Here's how the part is built. I have some questions about the finished solid (model axes, mm). Round coordinates to 2 decimals unless told otherwise and drop trailing zeros. Write each loop counter-clockwise with the first axis right and the second up, starting at its lowest first coordinate (ties: lowest second). Pieces come first, ordered by that corner, then holes. Notation, with made-up numbers: (78, 19) -> (116, 19) arc R24 cw to (116, 31) -> close; hole circle Ø10 at (71.25, -25.5). An arc over 180 degrees is marked (long way). Answer in a Markdown table with one row per item. Add a question column.
Autodesk Inventor part; units mm, degrees
ref_plane "att_plate_magnet_XY" through (19.5, -5, 7.5) normal (0, 0, 1) x (1, 0, 0)
ref_plane "att_plate_magnet_YZ" through (19.5, -5, 7.5) normal (1, 0, 0) x (0, 1, 0)
ref_plane "att_plate_magnet_ZX" through (19.5, -5, 7.5) normal (0, 1, 0) x (0, 0, 1)
sketch "Sketch_14" plane through (0, 0, 0) normal (0, 1, 0) x (-1, 0, 0)
  line L0 (25.5, 7.5) -> (-25.5, 7.5)
  line L1 (-25.5, 7.5) -> (-25.5, -7.5)
  line L2 (-25.5, -7.5) -> (25.5, -7.5)
  line L3 (25.5, -7.5) -> (25.5, 7.5)
  circle A0 centre (-15.5, -2.5) radius 2.75
  circle A1 centre (15.5, -2.5) radius 2.75
extrude "Extrusion1" add sketch "Sketch_14" along normal mid plane 20
sketch "Sketch_2" plane through (19.5, 0, 0) normal (1, 0, 0) x (0, 0, -1)
  line L0 (7.5, -5) -> (-7.5, -5)
  line L1 (-7.5, -5) -> (-7.5, -3)
  line L2 (-7.5, -3) -> (-7.121, -3.379)
  line L3 (-7.121, -3.379) -> (7.121, -3.379)
  line L4 (7.121, -3.379) -> (7.5, -3)
  line L5 (7.5, -3) -> (7.5, -5)
  line L6 (7.5, -5) -> (-7.5, -5)
revolve "Revolution1" cut sketch "Sketch_2" angle 360 about axis through (19.5, -5, -7.5) along (0, 0, -1)
thread "Thread1"
sketch "Sketch_3" plane through (-19.5, 0, 0) normal (1, 0, 0) x (0, 0, -1)
  line L0 (7.5, -5) -> (-7.5, -5)
  line L1 (-7.5, -5) -> (-7.5, -3)
  line L2 (-7.5, -3) -> (-7.121, -3.379)
  line L3 (-7.121, -3.379) -> (7.121, -3.379)
  line L4 (7.121, -3.379) -> (7.5, -3)
  line L5 (7.5, -3) -> (7.5, -5)
  line L6 (7.5, -5) -> (-7.5, -5)
revolve "Revolution2" cut sketch "Sketch_3" angle 360 about axis through (-19.5, -5, -7.5) along (0, 0, -1)
thread "Thread2"
ref_plane "att_plate_magnet_XY" through (19.5, -5, 7.5) normal (0, 0, 1) x (1, 0, 0)
ref_plane "att_plate_magnet_YZ" through (19.5, -5, 7.5) normal (1, 0, 0) x (0, 1, 0)
ref_plane "att_plate_magnet_ZX" through (19.5, -5, 7.5) normal (0, 1, 0) x (0, 0, 1)
ref_plane "to_magnetT_XY" through (-19.5, -5, 7.5) normal (0, 0, 1) x (1, 0, 0)
ref_plane "to_magnetT_YZ" through (-19.5, -5, 7.5) normal (1, 0, 0) x (0, 1, 0)
ref_plane "to_magnetT_ZX" through (-19.5, -5, 7.5) normal (0, 1, 0) x (0, 0, 1)
ref_plane "c1_XY" through (-15.5, 10, -2.5) normal (0, 1, 0) x (1, 0, 0)
ref_plane "c1_YZ" through (-15.5, 10, -2.5) normal (1, 0, 0) x (0, 0, -1)
ref_plane "c1_ZX" through (-15.5, 10, -2.5) normal (0, 0, -1) x (0, 1, 0)
ref_plane "c2_XY" through (15.5, 10, -2.5) normal (0, 1, 0) x (1, 0, 0)
ref_plane "c2_YZ" through (15.5, 10, -2.5) normal (1, 0, 0) x (0, 0, -1)
ref_plane "c2_ZX" through (15.5, 10, -2.5) normal (0, 0, -1) x (0, 1, 0)
ref_plane "c3_XY" through (-15.5, -10, -2.5) normal (0, 1, 0) x (1, 0, 0)
ref_plane "c3_YZ" through (-15.5, -10, -2.5) normal (1, 0, 0) x (0, 0, -1)
ref_plane "c3_ZX" through (-15.5, -10, -2.5) normal (0, 0, -1) x (0, 1, 0)
ref_plane "c4_XY" through (15.5, -10, -2.5) normal (0, 1, 0) x (1, 0, 0)
ref_plane "c4_YZ" through (15.5, -10, -2.5) normal (1, 0, 0) x (0, 0, -1)
ref_plane "c4_ZX" through (15.5, -10, -2.5) normal (0, 0, -1) x (0, 1, 0)
ref_plane "cc3_XY" through (-15.5, 10, -2.5) normal (0, 1, 0) x (1, 0, 0)
ref_plane "cc3_YZ" through (-15.5, 10, -2.5) normal (1, 0, 0) x (0, 0, -1)
ref_plane "cc3_ZX" through (-15.5, 10, -2.5) normal (0, 0, -1) x (0, 1, 0)
ref_plane "cc4_XY" through (15.5, 10, -2.5) normal (0, 1, 0) x (1, 0, 0)
ref_plane "cc4_YZ" through (15.5, 10, -2.5) normal (1, 0, 0) x (0, 0, -1)
ref_plane "cc4_ZX" through (15.5, 10, -2.5) normal (0, 0, -1) x (0, 1, 0)
ref_plane "cc1_XY" through (-15.5, -10, -2.5) normal (0, 1, 0) x (1, 0, 0)
ref_plane "cc1_YZ" through (-15.5, -10, -2.5) normal (1, 0, 0) x (0, 0, -1)
ref_plane "cc1_ZX" through (-15.5, -10, -2.5) normal (0, 0, -1) x (0, 1, 0)
ref_plane "cc2_XY" through (15.5, -10, -2.5) normal (0, 1, 0) x (1, 0, 0)
ref_plane "cc2_YZ" through (15.5, -10, -2.5) normal (1, 0, 0) x (0, 0, -1)
ref_plane "cc2_ZX" through (15.5, -10, -2.5) normal (0, 0, -1) x (0, 1, 0)
ref_plane "d1_XY" through (15.5, 15, -5) normal (0, 1, 0) x (1, 0, 0)
ref_plane "d1_YZ" through (15.5, 15, -5) normal (1, 0, 0) x (0, 0, -1)
ref_plane "d1_ZX" through (15.5, 15, -5) normal (0, 0, -1) x (0, 1, 0)
ref_plane "d2_XY" through (-15.5, 15, -5) normal (0, 1, 0) x (1, 0, 0)
ref_plane "d2_YZ" through (-15.5, 15, -5) normal (1, 0, 0) x (0, 0, -1)
ref_plane "d2_ZX" through (-15.5, 15, -5) normal (0, 0, -1) x (0, 1, 0)
ref_plane "e1_XY" through (-15.5, 15, -5) normal (0, 1, 0) x (1, 0, 0)
ref_plane "e1_YZ" through (-15.5, 15, -5) normal (1, 0, 0) x (0, 0, -1)
ref_plane "e1_ZX" through (-15.5, 15, -5) normal (0, 0, -1) x (0, 1, 0)
ref_plane "e2_XY" through (15.5, 15, -5) normal (0, 1, 0) x (1, 0, 0)
ref_plane "e2_YZ" through (15.5, 15, -5) normal (1, 0, 0) x (0, 0, -1)
ref_plane "e2_ZX" through (15.5, 15, -5) normal (0, 0, -1) x (0, 1, 0)
ref_plane "p1_XY" through (15.5, 10, 0) normal (0, 1, 0) x (1, 0, 0)
ref_plane "p1_YZ" through (15.5, 10, 0) normal (1, 0, 0) x (0, 0, -1)
ref_plane "p1_ZX" through (15.5, 10, 0) normal (0, 0, -1) x (0, 1, 0)
ref_plane "p2_XY" through (-15.5, 10, 0) normal (0, 1, 0) x (1, 0, 0)
ref_plane "p2_YZ" through (-15.5, 10, 0) normal (1, 0, 0) x (0, 0, -1)
ref_plane "p2_ZX" through (-15.5, 10, 0) normal (0, 0, -1) x (0, 1, 0)
ref_plane "xxxx_XY" through (0, 0, 0) normal (0, 0, 1) x (1, 0, 0)
ref_plane "xxxx_YZ" through (0, 0, 0) normal (1, 0, 0) x (0, 1, 0)
ref_plane "xxxx_ZX" through (0, 0, 0) normal (0, 1, 0) x (0, 0, 1)
ref_plane "p11_XY" through (15.5, 10, 31) normal (0, 1, 0) x (1, 0, 0)
ref_plane "p11_YZ" through (15.5, 10, 31) normal (1, 0, 0) x (0, 0, -1)
ref_plane "p11_ZX" through (15.5, 10, 31) normal (0, 0, -1) x (0, 1, 0)
ref_plane "p22_XY" through (-15.5, 10, 31) normal (0, 1, 0) x (1, 0, 0)
ref_plane "p22_YZ" through (-15.5, 10, 31) normal (1, 0, 0) x (0, 0, -1)
ref_plane "p22_ZX" through (-15.5, 10, 31) normal (0, 0, -1) x (0, 1, 0)
ref_plane "plate_to_magnet_XY" through (-19.5, -5, 7.5) normal (0, 1, 0) x (1, 0, 0)
ref_plane "plate_to_magnet_YZ" through (-19.5, -5, 7.5) normal (1, 0, 0) x (0, 0, -1)
ref_plane "plate_to_magnet_ZX" through (-19.5, -5, 7.5) normal (0, 0, -1) x (0, 1, 0)
properties part number "MG5-5-ap"
Item 1: If we section it at B-B on z = -0.25: Please give me the cut outline in (x, y), then the cut area to 3 significant figures.
Item 2: If we section it at A-A on x = -19.5: Please give me the cut outline in (y, z), then the cut area to 3 significant figures.
Item 3: If we mould it in two halves opening along Y, with no side actions, what happens to faces 1 (the cylindrical face through (-21.082, -5.351, -0.1)), 2 (the flat face through (-25.5, 0, 0)), 3 (the cylindrical face through (21.107, -5.211, -0.1)), 4 (the flat face through (0, -10, 0))? For each: pulls with the +Y half, pulls with the -Y half, needs draft (parallel to the pull), parting line crosses it, or undercut.
Item 4: I need wall thicknesses on line 1 along X through (y, z) = (6.5, -3.25); line 2 along X through (y, z) = (-4.5, -4.5); line 3 along Z through (x, y) = (15.5, 5.5). Which ranges of each line are inside material? Lowest first, please. Write a range as from..to.
Item 5: If we section it at C-C on y = -5: Please give me the cut outline in (x, z), then the cut area to 3 significant figures.
Item 6: If we section it at D-D on z = -3.5: Please give me the cut outline in (x, y), then the cut area to 3 significant figures.
Results list:
| question | item | result |
|---|---|---|
| 1 | outline | (-25.5, -10) -> (-17.08, -10) -> (-17.08, 10) -> (-25.5, 10) -> close; (-13.92, -10) -> (13.92, -10) -> (13.92, 10) -> (-13.92, 10) -> close; (17.08, -10) -> (25.5, -10) -> (25.5, 10) -> (17.08, 10) -> close; hole circle Ø3.24 at (-19.5, -5); hole circle Ø3.24 at (19.5, -5) |
| 1 | area | 877 mm² |
| 2 | outline | (-10, -7.5) -> (-7, -7.5) -> (-6.62, -7.12) -> (-6.62, 7.12) -> (-7, 7.5) -> (-10, 7.5) -> close; (-3.38, -7.12) -> (-3, -7.5) -> (10, -7.5) -> (10, 7.5) -> (-3, 7.5) -> (-3.38, 7.12) -> close |
| 2 | area | 251 mm² |
| 3 | face 1 | undercut |
| 3 | face 2 | needs draft |
| 3 | face 3 | undercut |
| 3 | face 4 | pulls with the -Y half |
| 4 | line 1 | -25.5..-18.15, -12.85..12.85, 18.15..25.5 |
| 4 | line 2 | -25.5..-21.04, -17.96..-17.39, -13.61..13.61, 17.39..17.96, 21.04..25.5 |
| 4 | line 3 | -7.5..-5.25, 0.25..7.5 |
| 5 | outline | (-25.5, -7.5) -> (-21.5, -7.5) -> (-21.12, -7.12) -> (-21.12, 7.12) -> (-21.5, 7.5) -> (-25.5, 7.5) -> close; (-17.88, -7.12) -> (-17.5, -7.5) -> (17.5, -7.5) -> (17.88, -7.12) -> (17.88, -3.88) arc R2.75 cw (long way) to (17.88, -1.12) -> (17.88, 7.12) -> (17.5, 7.5) -> (-17.5, 7.5) -> (-17.88, 7.12) -> (-17.88, -1.12) arc R2.75 cw (long way) to (-17.88, -3.88) -> close; (21.12, -7.12) -> (21.5, -7.5) -> (25.5, -7.5) -> (25.5, 7.5) -> (21.5, 7.5) -> (21.12, 7.12) -> close |
| 5 | area | 621 mm² |
| 6 | outline | (-25.5, -10) -> (-18.06, -10) -> (-18.06, -5.75) arc R1.62 cw (long way) to (-18.06, -4.25) -> (-18.06, 10) -> (-25.5, 10) -> close; (-12.94, -10) -> (12.94, -10) -> (12.94, 10) -> (-12.94, 10) -> close; (18.06, -10) -> (25.5, -10) -> (25.5, 10) -> (18.06, 10) -> (18.06, -4.25) arc R1.62 cw (long way) to (18.06, -5.75) -> close |
| 6 | area | 799 mm² |
